```python
from build123d import *

# Parameters (mm, degrees)
EXTRUDE_1_DEPTH          = 13
CUT_EXTRUDE_1_DEPTH      = 48.634021455
CUT_EXTRUDE_1_DEPTH_BACK = 48.634021455


with BuildPart() as part:
    # 草圖1 → 填料-伸長1 (new body)
    with BuildSketch(Plane(origin=(0, 0, 0), x_dir=(1, 0, 0), z_dir=(0, 1, 0))):
        Polygon((17.320508076, -30), (34.641016151, 0), (17.320508076, 30), (-17.320508076, 30), (-34.641016151, 0), (-17.320508076, -30), align=None)
    extrude(amount=EXTRUDE_1_DEPTH)

    # 草圖2 → 除料-伸長1 (cut, two sides: drawn at the far end of the back side and taken through both)
    with BuildSketch(Plane.XY.offset(-CUT_EXTRUDE_1_DEPTH_BACK)):
        Polygon((-12.5, 0), (-7.5, 0), (-5, 8), (-15, 8), align=None)
        Polygon((-34.641016151, 0), (-27.5, 0), (-25, 8), (-34.641016151, 8), align=None)
        Polygon((5, 8), (7.5, 0), (12.5, 0), (15, 8), align=None)
        Polygon((25, 8), (27.5, 0), (34.641016151, 0), (34.641016151, 8), align=None)
    extrude(amount=CUT_EXTRUDE_1_DEPTH + CUT_EXTRUDE_1_DEPTH_BACK, mode=Mode.SUBTRACT)

    # 草圖3 → 除料-旋轉1 (revolve, cut)
    with BuildSketch(Plane.XY, mode=Mode.PRIVATE) as cut_revolve_1_sk:
        Polygon((0, 10), (-22.5, 10), (-20, 0), (0, 0), align=None)
    revolve(cut_revolve_1_sk.sketch.rotate(Axis((0, 13.801022721, 0), (0, -1, 0)), 270), axis=Axis((0, 13.801022721, 0), (0, -1, 0)), mode=Mode.SUBTRACT)

    # 草圖4 → 除料-旋轉7 (revolve, cut)
    with BuildSketch(Plane.XY, mode=Mode.PRIVATE) as cut_revolve_7_sk:
        Polygon((34.641016151, 10), (34.641016151, 13), (29.641016151, 13), align=None)
    revolve(cut_revolve_7_sk.sketch.rotate(Axis((0, 13, 0), (0, -1, 0)), 180), axis=Axis((0, 13, 0), (0, -1, 0)), mode=Mode.SUBTRACT)


solid = part.part
```
Can you work these out from the model? Positions are in its coordinate system, mm. A direction names the side the tool comes from. Round coordinates to 2 decimals unless told otherwise and drop trailing zeros. Order: outer loops, then holes, each group sorted by start corner. A loop starts at its lowest first (then second) coordinate and runs counter-clockwise, first axis right, second up. Notation, with made-up numbers: (20, -24) -> (35, -24) arc R8 cw to (35, -9) -> close; hole circle Ø5 at (57.5, 16.5). An arc over 180 degrees is marked (long way). Return JSON: item names as keys, results as strings. Group by question number.
1. If we section it at C-C, the plane y = 9.25: Write out the boundary of the cut face in (x, z) (1 decimal), then the cut area to 3 significant figures.
2. Will these pins go through, and if not, where does the flat tip stop? pin 1 (1.5 mm diameter, centred on x = 23.5, z = -15.5, fed in from -Y); pin 2 (1 mm diameter, centred on y = 3, z = -9, fed in from -X); pin 3 (4 mm diameter, centred on x = 27, z = -17, fed in from +Y); pin 4 (1 mm diameter, centred on y = 9, z = -9, fed in from -X).
3. We'd pull the mould along X, two halves only. Please class faces 5 (the face through (-22, 0, 0)), 6 (the face through (10, 8, 24)), 7 (the face through (-23.935, 6.303, -18.543)), 8 (the face through (24.18, 6.3, -18.12)): released by +X, released by -X, zero draft, split by the parting line, or undercut.
4. I need wall thicknesses on line 1 (X direction, y = 9, z = -10); line 2 (Z direction, x = -8.5, y = 9); line 3 (Y direction, x = -29.5, z = 0). Which ranges of each line are inside material? Lowest first, please. Write a range as [from, to].
5. If we section it at B-B, the plane x = 0: Write out the boundary of the cut face in (y, z).
6. If we section it at A-A, the plane y = 3.75: Write out the boundary of the cut face in (x, z) (1 decimal), then the cut area to 3 significant figures.
7. Which directions (+Z, -Z, +X, -X, +Y, -Y) give clear straight access to the entire face, cutting with the end or side of a thin tool? Please do faces 1 (the face through (0, 10, 0)), 2 (the face through (-29, 8, 0)), 3 (the face through (13.73, 3.94, -22.91)), 4 (the face through (0, 0, -24)).
Output values:
{
 "1": {"outline": "(-34.6, 0) -> (-17.3, -30) -> (17.3, -30) -> (34.6, 0) -> (17.3, 30) -> (-17.3, 30) -> close; hole circle Ø44.6 at (0, 0)", "area": "1,550 mm²"},
 "2": {"pin 1": "y = 0", "pin 2": "x = -26.72", "pin 3": "y = 12.84", "pin 4": "x = -29.73"},
 "3": {"face 5": "zero draft", "face 6": "undercut", "face 7": "released by -X", "face 8": "released by +X"},
 "4": {"line 1": "[-28.87, -19.88], [19.88, 28.87]", "line 2": "[-30, -20.56], [20.56, 30]", "line 3": "[8, 13]"},
 "5": {"outline": "(0, -30) -> (12.78, -30) -> (13, -29.64) -> (13, 29.64) -> (12.78, 30) -> (0, 30) -> (0, 20) -> (10, 22.5) -> (10, -22.5) -> (0, -20) -> close"},
 "6": {"outline": "(-26.3, -14.4) -> (-17.3, -30) -> (-13.7, -30) -> (-13.7, -15.9) arc R20.9 cw to (-13.7, 15.9) -> (-13.7, 30) -> (-17.3, 30) -> (-26.3, 14.4) -> close; (-6.3, -30) -> (6.3, -30) -> (6.3, -20) arc R20.9 cw to (-6.3, -20) -> close; (-6.3, 20) arc R20.9 cw to (6.3, 20) -> (6.3, 30) -> (-6.3, 30) -> close; (13.7, -30) -> (17.3, -30) -> (26.3, -14.4) -> (26.3, 14.4) -> (17.3, 30) -> (13.7, 30) -> (13.7, 15.9) arc R20.9 cw to (13.7, -15.9) -> close", "area": "1,160 mm²"},
 "7": {"face 1": "none", "face 2": "+Z, -Z, -X", "face 3": "+Z, -Z", "face 4": "+Z, -Z, +X, -X, -Y"}
}
